Could you check a few things on this model? Use its own coordinates, in mm. Face numbers are marked on the shaded views. A direction names the side the tool comes from. Give positions to 0.01 mm unless a question says otherwise; leave off trailing zeros. Order: outer loops, then holes, each group sorted by start corner. A loop starts at its lowest first (then second) coordinate and runs counter-clockwise, first axis right, second up.
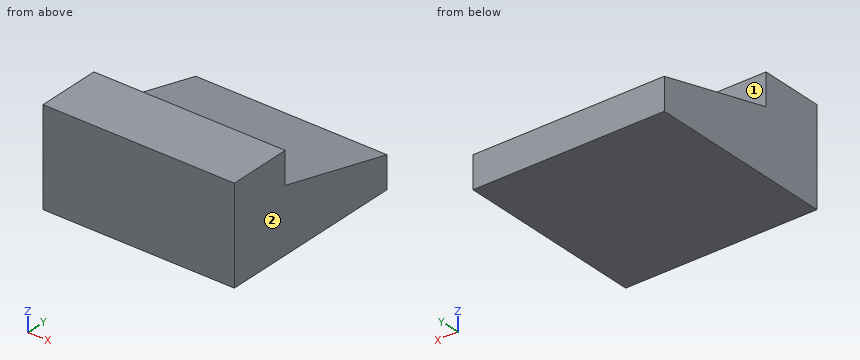
from build123d import *

# Parameters (mm, degrees)
F0_W     = 30
F0_H     = 30
F1_DEPTH = 15
F3_DEPTH = 30.001


with BuildPart() as f1:
    # F0 (on Top) → F1 (new body)
    with BuildSketch(Plane.XY):
        with Locations((-31.776512, 32.623932)):
            Rectangle(F0_W, F0_H)
    extrude(amount=F1_DEPTH)

    # F2 (on face) → F3 (cut, through all)
    with BuildSketch(Plane.YZ.offset(-16.776512)):
        Polygon((27.623932, 10), (47.623932, 5), (47.623932, 15), (27.623932, 15), align=None)
    extrude(amount=-F3_DEPTH, mode=Mode.SUBTRACT)


solid = f1.part
Item 1: For pin 1 (1.5 mm diameter, centred on x = -26.5, z = 13.5, fed in from +Y), with a flat end and sliding along its axis, tell me the tip position at first contact or that it passes through.
Findings:
pin 1: stops at y = 27.62
Item 2: Imagine slicing it at C-C on y = 42. List the corners of the cut face in (x, z) for me.
Findings:
outline: (-46.78, 0) - (-16.78, 0) - (-16.78, 6.41) - (-46.78, 6.41) - close
Item 3: For the marked faces 1 and 2, which set-ups out of +Z, -Z, +X, -X, +Y, -Y let a thin tool reach every point of the face, with its end or its side?
Findings:
face 1: +Z, +X, -X, +Y
face 2: +Z, -Z, +X, +Y, -Y
Item 4: Imagine slicing it at B-B on z = 12.25. List the corners of the cut face in (x, y) for me, then the cut area to 3 significant figures.
Findings:
outline: (-46.78, 17.62) - (-16.78, 17.62) - (-16.78, 27.62) - (-46.78, 27.62) - close
area: 300 mm2
Item 5: Please list where these lines run through material, in increasing order: line 1 along Y through (x, z) = (-23.25, 13.75); line 2 along Z through (x, y) = (-33.75, 35); line 3 along Z through (x, y) = (-33, 34).
Findings:
line 1: y = 17.62 to 27.62
line 2: z = 0 to 8.16
line 3: z = 0 to 8.41
Item 6: Imagine slicing it at A-A on x = -39.5. List the corners of the cut face in (y, z) for me, then the cut area to 3 significant figures.
Findings:
outline: (17.62, 0) - (47.62, 0) - (47.62, 5) - (27.62, 10) - (27.62, 15) - (17.62, 15) - close
area: 300 mm2
